For this review, use the dimensioned drawing (mm, ordinates from the lowest corner) and the shaded views. Give positions to 0.01 mm unless a question says otherwise; leave off trailing zeros. Loops run counter-clockwise (first coordinate to the right, second up) from the corner with the lowest first, then second, coordinate; pieces in that order, holes last. Notation, with made-up numbers: (76, 61) -> (105, 61) arc R17 ccw to (105, 75) -> close; hole circle Ø5 at (4, 63.5). An arc over 180 degrees is marked (long way). Use a Markdown table: item, result. Add a question column.
1. Add section A-A (x = 6.6). State the section outline as (y, z) points.
2. For pin 1 Ø2 at (x, z) = (4, 9) entering from -Y, flat-tipped, find the tip position at first contact; note if it passes through.
3. To check wall thickness, follow line 1 (Y direction, x = 6.6, z = 3.95). State the ranges of the line that lie inside material, in increasing order.
4. Draft analysis for pull direction Y (two halves, no side actions). For the marked faces 1, 2 and 3, state which applies: pulls with the +Y half, pulls with the -Y half, needs draft (parallel to the pull), parting line crosses it, or undercut.
5. Add section C-C (y = 9.25). State the section outline as (x, z) points.
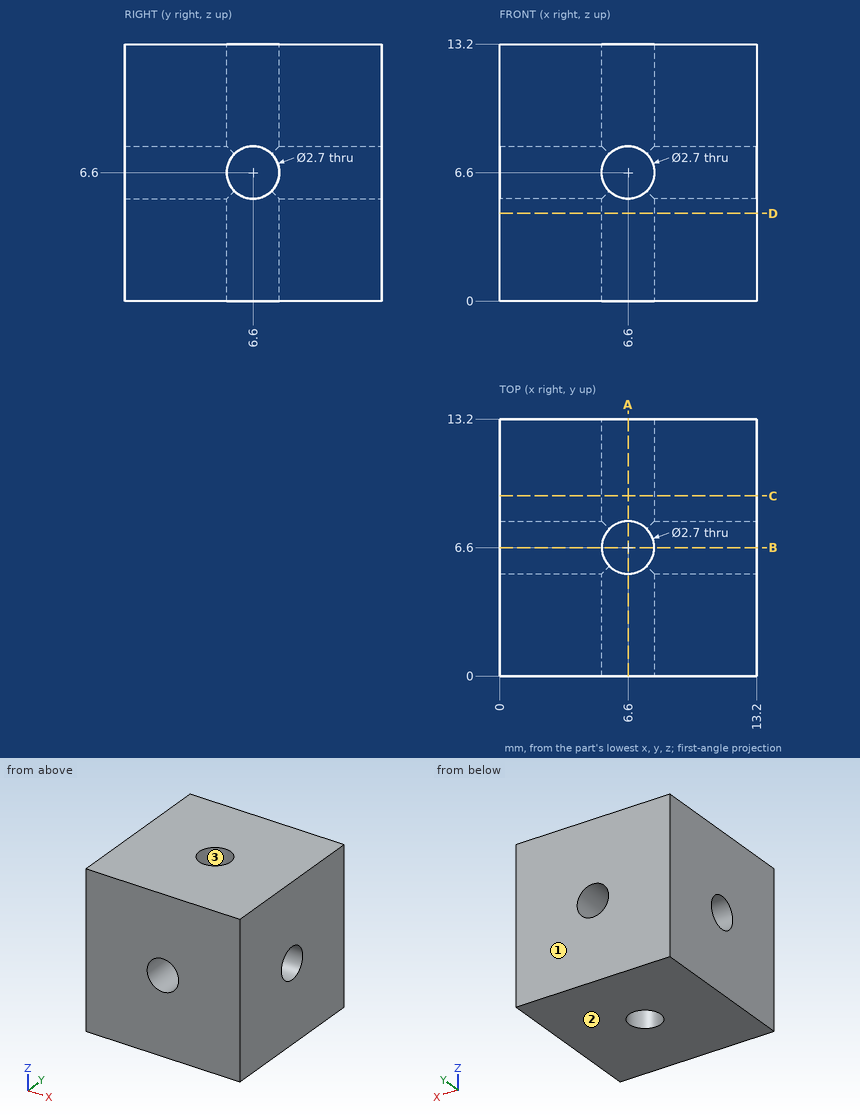
Taken from the geometry:
| question | item | result |
|---|---|---|
| 1 | outline | (0, 0) -> (5.25, 0) -> (5.25, 5.25) -> (0, 5.25) -> close; (0, 7.95) -> (5.25, 7.95) -> (5.25, 13.2) -> (0, 13.2) -> close; (7.95, 0) -> (13.2, 0) -> (13.2, 5.25) -> (7.95, 5.25) -> close; (7.95, 7.95) -> (13.2, 7.95) -> (13.2, 13.2) -> (7.95, 13.2) -> close |
| 2 | pin 1 | stops at y = 0 |
| 3 | line 1 | y = 0 to 5.25, 7.95 to 13.2 |
| 4 | face 1 | pulls with the +Y half |
| 4 | face 2 | needs draft |
| 4 | face 3 | undercut |
| 5 | outline | (0, 0) -> (13.2, 0) -> (13.2, 13.2) -> (0, 13.2) -> close; hole circle Ø2.7 at (6.6, 6.6) |
